Could you check a few things on this drawing? It's one solid part, dimensions in mm from its lowest x, y, z. A direction names the side the tool comes from. Give positions to 0.01 mm unless a question says otherwise; leave off trailing zeros. Order: outer loops, then holes, each group sorted by start corner. A loop starts at its lowest first (then second) coordinate and runs counter-clockwise, first axis right, second up. Notation, with made-up numbers: M -10.75,44 L 21.25,44 A24 ccw 21.25,77 Z; hole C 54,52 d1. An arc over 180 degrees is marked long. One line per item, written item: value. Start each with the question number.
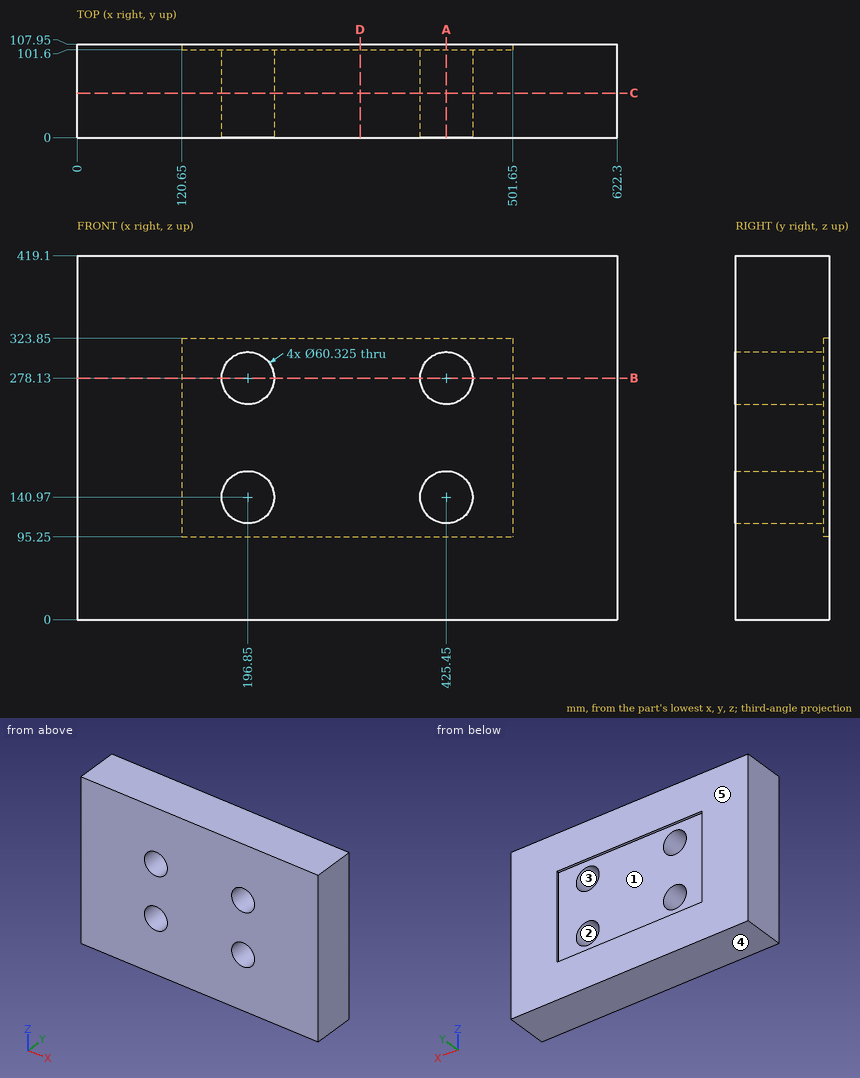
Item 1: I want a section at D-D on x = 326. Write out the boundary of the cut face in (y, z).
Item 2: I want a section at C-C on y = 51.5. Count the separate pieces of the cut face and the enclosed holes in it, plus the area to 3 significant figures.
Item 3: We'd pull the mould along Z, two halves only. Please class the marked faces 3, 4 and 5: +Z half, -Z half, draft (parallel to the pull), parting line (faces both ways), or undercut.
Item 4: Will this pin go through, and if not, where does the flat tip stop? P1, Ø7, axis at x = 314, y = 105, coming from the -Z side.
Item 5: For the marked faces 1 and 2, which set-ups out of +Z, -Z, +X, -X, +Y, -Y let a thin tool reach every point of the face, with its end or its side?
Item 6: I want a section at B-B on z = 278.13. Write out the boundary of the cut face in (x, y), plus the area to 3 significant figures.
Item 7: I want a section at A-A on x = 425.45. Write out the boundary of the cut face in (y, z), plus the area to 3 significant figures.
Item 8: Please list where these lines run through material, in increasing order: probe 1 along X at (y, z) = (45, 140); probe 2 along Z at (x, y) = (196.85, 24); probe 3 along X at (y, z) = (32.5, 138). Write a range as [from, to].
Answer below:
1. outline: M 0,0 L 107.95,0 L 107.95,95.25 L 101.6,95.25 L 101.6,323.85 L 107.95,323.85 L 107.95,419.1 L 0,419.1 Z
2. separate pieces: 1
2. enclosed holes: 4
2. area: 249,000 mm²
3. face 3: undercut
3. face 4: -Z half
3. face 5: draft
4. P1: stops at z = 0
5. face 1: +Y
5. face 2: +Y, -Y
6. outline: M 0,0 L 166.69,0 L 166.69,101.6 L 120.65,101.6 L 120.65,107.95 L 0,107.95 Z; M 227.01,0 L 395.29,0 L 395.29,101.6 L 227.01,101.6 Z; M 455.61,0 L 622.3,0 L 622.3,107.95 L 501.65,107.95 L 501.65,101.6 L 455.61,101.6 Z
6. area: 52,500 mm²
7. outline: M 0,0 L 107.95,0 L 107.95,95.25 L 101.6,95.25 L 101.6,110.81 L 0,110.81 Z; M 0,171.13 L 101.6,171.13 L 101.6,247.97 L 0,247.97 Z; M 0,308.29 L 101.6,308.29 L 101.6,323.85 L 107.95,323.85 L 107.95,419.1 L 0,419.1 Z
7. area: 31,500 mm²
8. probe 1: x = [0, 166.7], [227, 395.3], [455.6, 622.3]
8. probe 2: z = [0, 110.81], [171.13, 247.97], [308.29, 419.1]
8. probe 3: x = [0, 166.83], [226.87, 395.43], [455.47, 622.3]
